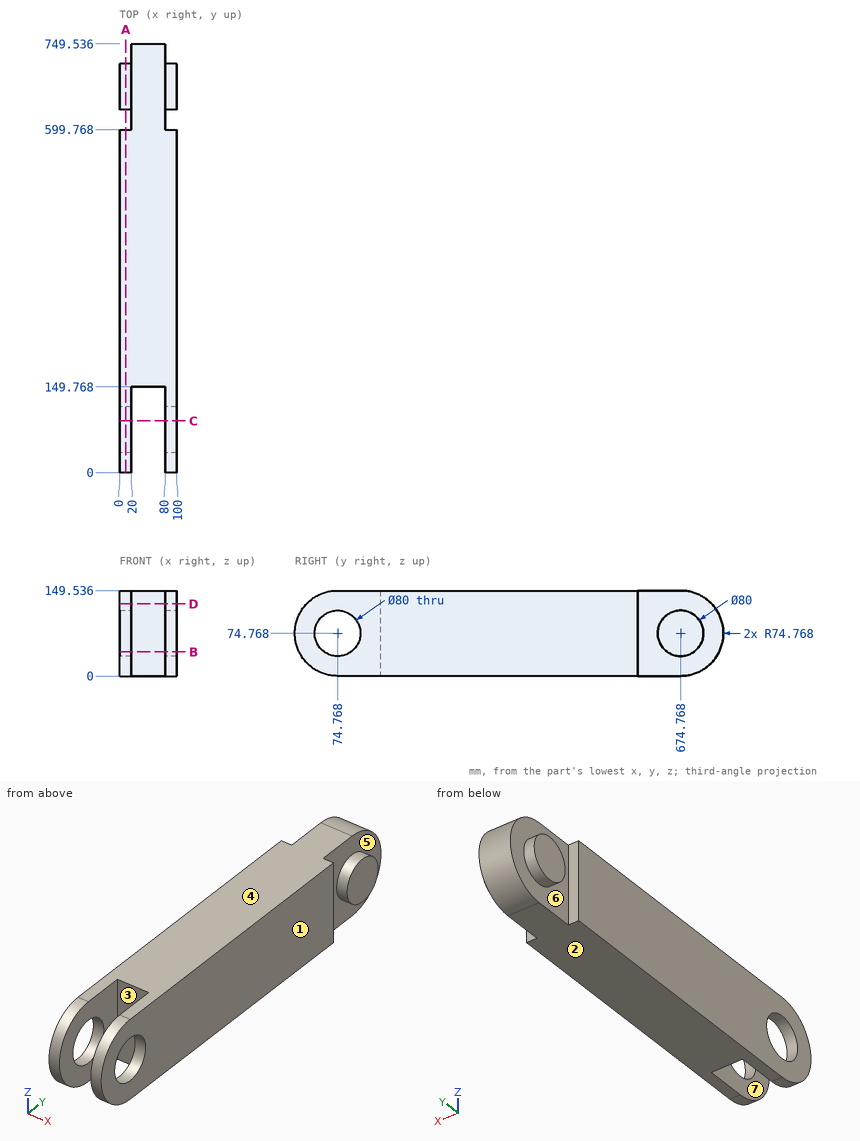
Print and shaded views of the part. All mm, measured from the part's lowest x, y and z. A direction names the side the tool comes from. Coordinates: 2 decimals unless noted, no trailing zeros. Write each loop counter-clockwise with the first axis right and the second up, starting at its lowest first coordinate (ties: lowest second). Pieces come first, ordered by that corner, then holes.
(1) Cut at D-D, the plane z = 126. List the corners of the cut face in (x, y).
(2) Cut at B-B, the plane z = 42. List the corners of the cut face in (x, y).
(3) Two-plate mould, pull along X, no slides. Class the marked faces 1, 2 and 3: +X half, -X half, draft (parallel to the pull), parting line (faces both ways), or undercut.
(4) Cut at C-C, the plane y = 90.5. List the corners of the cut face in (x, z) (1 decimal).
(5) 3-axis set-ups, long thin cutter, end or side, ignore diameter. For the marked faces 4, 5, 6 and 7: which of +Z, -Z, +X, -X, +Y, -Y reach the whole face in a straight line?
(6) Drill centre lines: probe 1 along Y at (x, z) = (12, 87) (1 decimal); probe 2 along Y at (x, z) = (16.5, 70); probe 3 along Y at (x, z) = (88, 30.5) (1 decimal). Where is each one in solid material? Low to high.
(7) Cut at A-A, the plane x = 11. List the corners of the cut face in (y, z) (1 decimal), and give its area (3 significant figures).
(8) Flat gauge pins, fed straight in: pin 1 (3 mm diameter, centred on x = 31.5, z = 17.5, fed in from +Y); pin 2 (1.5 mm diameter, centred on x = 15, z = 108, fed in from -Y) (1 decimal); pin 3 (6 mm diameter, centred on x = 11.5, z = 55, fed in from +Y). Where does each tip first touch, or does it go through?
Geometry says:
1. outline: (0, 20.31) - (20, 20.31) - (20, 149.77) - (80, 149.77) - (80, 20.31) - (100, 20.31) - (100, 599.77) - (80, 599.77) - (80, 729.22) - (20, 729.22) - (20, 599.77) - (0, 599.77) - close
2. outline: (0, 7.56) - (20, 7.56) - (20, 51.83) - (0, 51.83) - close; (0, 97.71) - (20, 97.71) - (20, 149.77) - (80, 149.77) - (80, 97.71) - (100, 97.71) - (100, 599.77) - (80, 599.77) - (80, 651.83) - (100, 651.83) - (100, 697.71) - (80, 697.71) - (80, 741.97) - (20, 741.97) - (20, 697.71) - (0, 697.71) - (0, 651.83) - (20, 651.83) - (20, 599.77) - (0, 599.77) - close; (80, 7.56) - (100, 7.56) - (100, 51.83) - (80, 51.83) - close
3. face 1: +X half
3. face 2: draft
3. face 3: undercut
4. outline: (0, 0) - (20, 0) - (20, 38) - (0, 38) - close; (0, 111.5) - (20, 111.5) - (20, 149.5) - (0, 149.5) - close; (80, 0) - (100, 0) - (100, 38) - (80, 38) - close; (80, 111.5) - (100, 111.5) - (100, 149.5) - (80, 149.5) - close
5. face 4: +Z, +X, -X, +Y, -Y
5. face 5: +X
5. face 6: -X
5. face 7: +Z, -Z, -Y
6. probe 1: y = 1 to 36.7, 112.9 to 599.8, 636.7 to 712.9
6. probe 2: y = 0.15 to 35.05, 114.48 to 599.77, 635.05 to 714.48
6. probe 3: y = 14.5 to 599.8
7. outline: (74.8, 0) - (599.8, 0) - (599.8, 149.5) - (74.8, 149.5) arc R74.8 ccw to start; circle Ø80 at (674.8, 74.8); hole circle Ø80 at (74.8, 74.8)
7. area: 87,300 mm2
8. pin 1: stops at y = 724.57
8. pin 2: stops at y = 7.4
8. pin 3: stops at y = 711.08
